Read the model definition and answer for the solid it produces. Units are mm, in the model's axes. A direction names the side the tool comes from. Coordinates: 2 decimals unless noted, no trailing zeros. Order: outer loops, then holes, each group sorted by start corner. A loop starts at its lowest first (then second) coordinate and runs counter-clockwise, first axis right, second up. Notation, with made-up numbers: M 88,50.25 L 129,50.25 A21 cw 129,70.25 Z; hole C -20.5,16 d3. An arc over 180 degrees is marked long. Use a Markdown table: item, result. Add a question column.
1) Find section B-B on y = 6. Write down the section's boundary in (x, z), plus the area to 3 significant figures.
2) Find section C-C on y = -32. Write down the section's boundary in (x, z), plus the area to 3 significant figures.
3) Find section A-A on z = 9. Write down the section's boundary in (x, y), plus the area to 3 significant figures.
4) Each of these flat-tipped pins is pushed along its axis until it touches: pin 1 Ø6 at (y, z) = (-21.5, 52) entering from +X; pin 2 Ø1 at (y, z) = (-14.5, 25.5) entering from -X; pin 3 Ø10.5 at (y, z) = (-19, 30.5) entering from -X. Where does it stop, or does it pass through?
5) Find the intervals of material crossed by probe 1 along Z at (x, y) = (-29.5, -30); probe 2 along Z at (x, y) = (80, -24.5); probe 3 along Y at (x, z) = (20.5, 61) (3 decimals), in increasing order. Write a range as [from, to].
6) For faces 1 (the face through (51, 25.4, 56)), 2 (the face through (48.26, -1, 5)), 3 (the face through (-4, 0, 43)), 4 (the face through (51, -25.4, 56)), 5 (the face through (39.206, -20.704, 68.649)), determine the directions among +Z, -Z, +X, -X, +Y, -Y from which every point of the face is accessible in a straight line to the end or side of a thin tool.
from build123d import *

# Parameters (mm, degrees)
F1_DEPTH = 63.5
F2_DEPTH = 25.4
F3_DEPTH = 15.875
F4_R     = 6.35


with BuildPart() as f1:
    # F0 (on Front) → F1 (new body, symmetric)
    with BuildSketch(Plane.XZ):
        Polygon((29.21, 19.05), (-48.26, 19.05), (-48.26, -19.05), (48.26, -19.05), (48.26, 19.05), align=None)
    extrude(amount=F1_DEPTH, both=True)

    # F0 (on Front) → F2 (join, symmetric)
    with BuildSketch(Plane.XZ):
        with BuildLine():
            Line((29.21, 44.45), (29.21, 19.05))
            Line((29.21, 19.05), (48.26, 19.05))
            Line((48.26, 19.05), (48.26, 44.45))
            ThreePointArc((48.26, 44.45), (52.418442, 54.912154), (62.624393, 59.664825))
            Line((62.624393, 59.664825), (62.624393, 78.728819))
            ThreePointArc((62.624393, 78.728819), (38.945686, 68.385116), (29.21, 44.45))
        make_face()
        with BuildLine():
            ThreePointArc((63.5, 78.74), (63.062161, 78.737205), (62.624393, 78.728819))
            Line((62.624393, 78.728819), (62.624393, 59.664825))
            ThreePointArc((62.624393, 59.664825), (63.062016, 59.683705), (63.5, 59.69))
            Line((63.5, 59.69), (85.484393, 59.69))
            Line((85.484393, 59.69), (85.484393, 78.74))
            Line((85.484393, 78.74), (63.5, 78.74))
        make_face()
    extrude(amount=F2_DEPTH, both=True)

    # F0 (on Front) → F3 (join)
    with BuildSketch(Plane.XZ):
        with BuildLine():
            add(Edge.make_bspline(
                [(-48.26, 19.05), (-35.762786, 48.370969), (14.062008, 80.255039), (62.624393, 78.770398)],
                knots=[0, 0, 0, 0, 125.944125, 125.944125, 125.944125, 125.944125], degree=3))
            Line((-48.26, 19.05), (29.21, 19.05))
            Line((29.21, 19.05), (29.21, 44.45))
            ThreePointArc((29.21, 44.45), (38.945686, 68.385116), (62.624393, 78.728819))
            Line((62.624393, 78.728819), (62.624393, 78.770398))
        make_face()
    extrude(amount=F3_DEPTH)

    # F4
    f4_edges = [f1.edges().sort_by_distance(p)[0] for p in [
        (48.26, -63.5, 0),
        (-48.26, -63.5, 0),
        (48.26, 63.5, 0),
        (-48.26, 63.5, 0),
    ]]
    fillet(f4_edges, radius=F4_R)


solid = f1.part
Check result:
| question | item | result |
|---|---|---|
| 1 | outline | M -48.26,-19.05 L 48.26,-19.05 L 48.26,44.45 A15.24 cw 62.62,59.66 A15.24 cw 63.5,59.69 L 85.48,59.69 L 85.48,78.74 L 63.5,78.74 A34.29 ccw 62.62,78.73 A34.29 ccw 29.21,44.45 L 29.21,19.05 L -48.26,19.05 Z |
| 1 | area | 5,320 mm2 |
| 2 | outline | M -48.26,-19.05 L 48.26,-19.05 L 48.26,19.05 L -48.26,19.05 Z |
| 2 | area | 3,680 mm2 |
| 3 | outline | M -48.26,-57.15 A6.35 ccw -41.91,-63.5 L 41.91,-63.5 A6.35 ccw 48.26,-57.15 L 48.26,57.15 A6.35 ccw 41.91,63.5 L -41.91,63.5 A6.35 ccw -48.26,57.15 Z |
| 3 | area | 12,200 mm2 |
| 4 | pin 1 | stops at x = 52.5 |
| 4 | pin 2 | stops at x = -45.24 |
| 4 | pin 3 | stops at x = -44.46 |
| 5 | probe 1 | z = [-19.05, 19.05] |
| 5 | probe 2 | z = [59.69, 78.74] |
| 5 | probe 3 | y = [-15.875, 0] |
| 6 | face 1 | +Z, +X, -X, +Y |
| 6 | face 2 | -Z, +X, +Y, -Y |
| 6 | face 3 | +Z, -X, +Y |
| 6 | face 4 | +Z, +X, -X, -Y |
| 6 | face 5 | +Z, -X, -Y |
